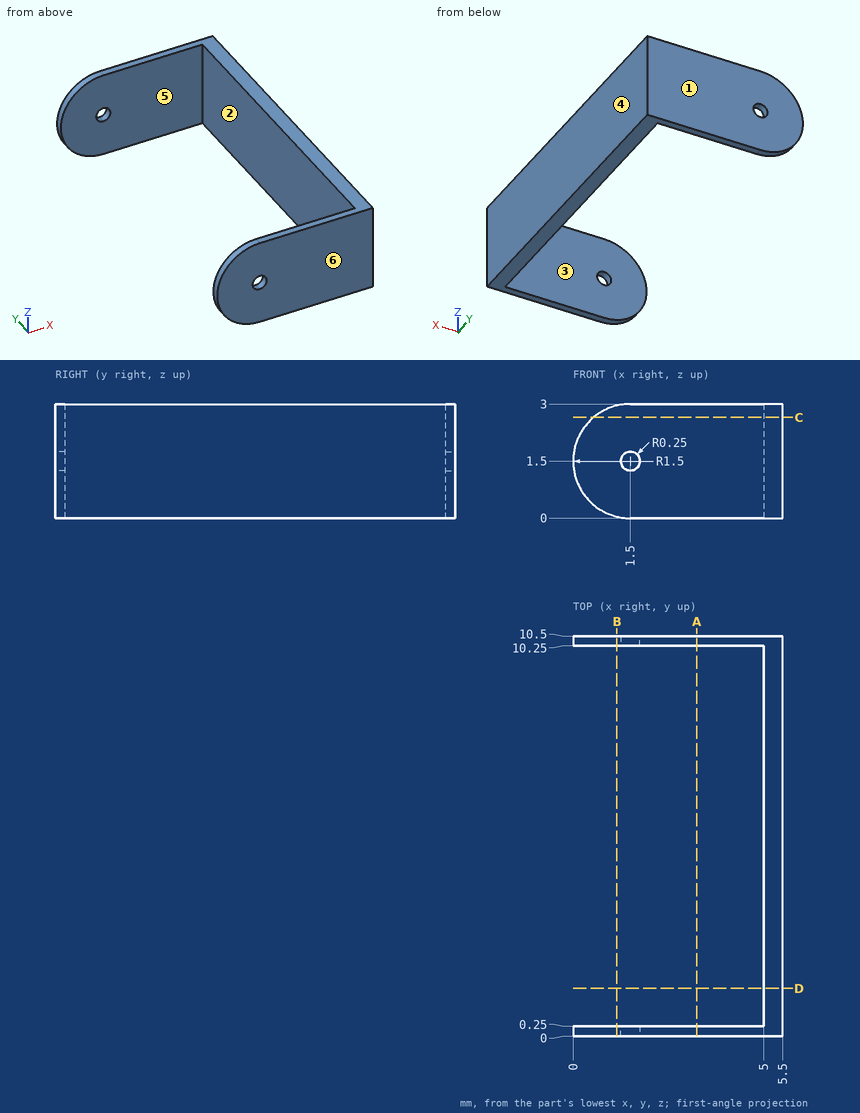
The figure shows three views and two pictorial views of one solid part (mm, origin at its lowest corner). Answer the questions. A direction names the side the tool comes from. Round coordinates to 2 decimals unless told otherwise and drop trailing zeros. Loops run counter-clockwise (first coordinate to the right, second up) from the corner with the lowest first, then second, coordinate; pieces in that order, holes last. Notation, with made-up numbers: M 13.25,59 L 32.25,59 A26 ccw 32.25,89 Z; hole C -5,39 d10. An arc over 180 degrees is marked long. Write each question's results on one line, items separated by ' | '. Start each with the question number.
1) Straight lines are drawn through the part: probe 1 along Y at (x, z) = (2.25, 0.5); probe 2 along X at (y, z) = (9.25, 1.85). For each, find the intervals that lie inside material, in ascending order.
2) Find section B-B on x = 1.15. Write down the section's boundary in (y, z).
3) Find section A-A on x = 3.25. Write down the section's boundary in (y, z).
4) Find section C-C on z = 2.65. Write down the section's boundary in (x, y).
5) Find section D-D on y = 1.25. Write down the section's boundary in (x, z).
6) This flat-tipped pin is pushed along its axis until it touches: pin 1 (0.9 mm diameter, centred on y = 5, z = 1, fed in from -X). Where does it stop, or does it pass through?
7) Determine the mould class of the marked faces 1, 2, 3 and 4 for opening direction Y: pulls with the +Y half, pulls with the -Y half, needs draft (parallel to the pull), parting line crosses it, or undercut.
8) Which of the six approach directions +Z, -Z, +X, -X, +Y, -Y give full straight-line access (tool end or side, diameter ignored) to the marked faces 5 and 6?
Final values:
1) probe 1: 0 to 0.25, 10.25 to 10.5 | probe 2: 5 to 5.5
2) outline: M 0,0.04 L 0.25,0.04 L 0.25,2.96 L 0,2.96 Z; M 10.25,0.04 L 10.5,0.04 L 10.5,2.96 L 10.25,2.96 Z
3) outline: M 0,0 L 0.25,0 L 0.25,3 L 0,3 Z; M 10.25,0 L 10.5,0 L 10.5,3 L 10.25,3 Z
4) outline: M 0.54,0 L 5.5,0 L 5.5,10.5 L 0.54,10.5 L 0.54,10.25 L 5,10.25 L 5,0.25 L 0.54,0.25 Z
5) outline: M 5,0 L 5.5,0 L 5.5,3 L 5,3 Z
6) pin 1: x = 5
7) face 1: pulls with the +Y half | face 2: undercut | face 3: undercut | face 4: needs draft
8) face 5: +Z, -Z, -X | face 6: +Z, -Z, +X, -X, -Y
